Read the model definition and answer for the solid it produces. Units are mm, in the model's axes. Face numbers are marked on the shaded views. A direction names the side the tool comes from. Coordinates: 2 decimals unless noted, no trailing zeros. Order: outer loops, then holes, each group sorted by start corner. A loop starts at its lowest first (then second) coordinate and runs counter-clockwise, first axis right, second up. Notation, with made-up numbers: (23, 35.25) - (74, 35.25) arc R8 cw to (74, 49.25) - close; hole circle Ø1 at (-31, -38). An arc over 180 degrees is marked (long way). Use one line per item in the form item = value. Start each with the question number.
from build123d import *

# Parameters (mm, degrees)
BOSS_EXTRUDE1_DEPTH = 75
SKETCH4_W           = 40
SKETCH4_H           = 50
CUT_EXTRUDE1_DEPTH  = 50
SKETCH5_R           = 12.5
CUT_EXTRUDE2_DEPTH  = 25


with BuildPart() as part:
    # Sketch2 → Boss-Extrude1 (new body)
    with BuildSketch(Plane.XY):
        Polygon((0, 0), (-65, 0), (-65, 50), (-150, 50), (-150, 75), (0, 75), align=None)
    extrude(amount=BOSS_EXTRUDE1_DEPTH)

    # Sketch4 → Cut-Extrude1 (cut)
    with BuildSketch(Plane.XY.offset(75)):
        with Locations((-20, 50)):
            Rectangle(SKETCH4_W, SKETCH4_H)
    extrude(amount=-CUT_EXTRUDE1_DEPTH, mode=Mode.SUBTRACT)

    # Sketch5 → Cut-Extrude2 (cut)
    with BuildSketch(Plane(origin=(0, 75, 0), x_dir=(1, 0, 0), z_dir=(0, 1, 0))):
        with Locations(Location((-115, -37.5, 0), (0, 0, 180))):
            Circle(SKETCH5_R)
    extrude(amount=-CUT_EXTRUDE2_DEPTH, mode=Mode.SUBTRACT)


solid = part.part
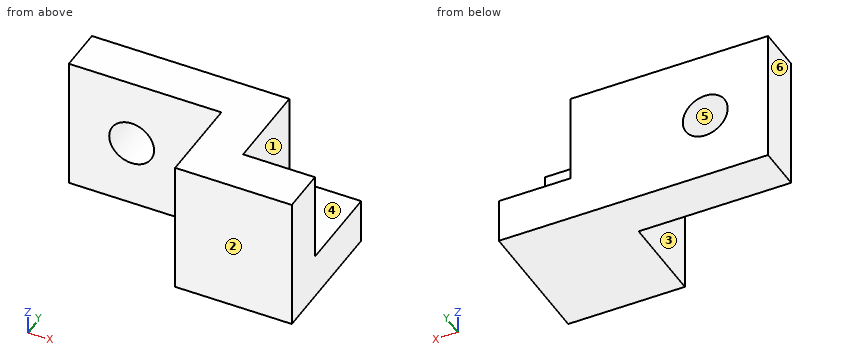
Q1. A cutting plane is placed at D-D (z = 62.5). Give the vertices of the cut face in (x, y), then the cut area to 3 significant figures.
Q2. Consider probe 1 along Z at (x, y) = (-115, 62); probe 2 along X at (y, z) = (14, 17); probe 3 along Y at (x, z) = (-94, 41). Determine where each line is inside the solid, lowest interval first.
Q3. For a pull along X with two mould halves and no side action, classify the marked faces 4, 5 and 6 as +X half, -X half, draft (parallel to the pull), parting line (faces both ways), or undercut.
Q4. A cutting plane is placed at A-A (z = 37.5). Give the vertices of the cut face in (x, y).
Q5. Given P1, Ø6, axis at y = 48.5, z = 37, coming from the +X side; P2, Ø8, axis at y = 42.5, z = 13.5, coming from the -X side; P3, Ø12, axis at x = -14.5, y = 59.5, coming from the +Z side, each flat-ended and moving along its own axis, determine where each tip first touches the part or whether it passes through.
Q6. A cutting plane is placed at C-C (x = -115). Give the vertices of the cut face in (y, z), then the cut area to 3 significant figures.
Q7. A cutting plane is placed at B-B (y = 55). Give the vertices of the cut face in (x, z), then the cut area to 3 significant figures.
Q8. Which of the six approach directions +Z, -Z, +X, -X, +Y, -Y give full straight-line access (tool end or side, diameter ignored) to the marked faces 1, 2 and 3?
Result sheet:
q1.outline = (-150, 50) - (-65, 50) - (-65, 0) - (0, 0) - (0, 25) - (-40, 25) - (-40, 75) - (-150, 75) - close
q1.area = 5,000 mm^2
q2.probe_1 = 0 to 25, 50 to 75
q2.probe_2 = -65 to 0
q2.probe_3 = 50 to 75
q3.face_4 = draft
q3.face_5 = undercut
q3.face_6 = -X half
q4.outline = (-150, 50) - (-127.5, 50) - (-127.5, 75) - (-150, 75) - close; (-102.5, 50) - (-65, 50) - (-65, 0) - (0, 0) - (0, 25) - (-40, 25) - (-40, 75) - (-102.5, 75) - close
q5.P1 = -40
q5.P2 = -65
q5.P3 = 25
q6.outline = (50, 0) - (75, 0) - (75, 25) - (50, 25) - close; (50, 50) - (75, 50) - (75, 75) - (50, 75) - close
q6.area = 1,250 mm^2
q7.outline = (-150, 0) - (0, 0) - (0, 25) - (-40, 25) - (-40, 75) - (-150, 75) - close; hole circle Ø25 at (-115, 37.5)
q7.area = 8,760 mm^2
q8.face_1 = +Z, +X, +Y
q8.face_2 = +Z, -Z, +X, -X, -Y
q8.face_3 = +Z, -Z, -X, -Y
